```python
from build123d import *

# Parameters (mm, degrees)
EXTRUDE_1_DEPTH     = 4
SKETCH_2_R          = 1.1
CUT_EXTRUDE_1_DEPTH = 4
SKETCH_3_R          = 1.1
CUT_EXTRUDE_2_DEPTH = 5
FILLET_3_R          = 1


with BuildPart() as part:
    # 草图1 → 凸台-拉伸1 (new body)
    with BuildSketch(Plane(origin=(0, 0, 0), x_dir=(1, 0, 0), z_dir=(0, 1, 0))):
        with BuildLine():
            Line((-6.657117104, 10.234542642), (-6.657117104, 3.551431113))
            Line((-6.657117104, 3.551431113), (-4.657117104, 3.551431113))
            Line((-4.657117104, 3.551431113), (-4.657117104, 11.058134514))
            ThreePointArc((-4.657117104, 11.058134514), (-4.457117104, 16.10020126), (-4.257117104, 11.058134514))
            Line((-4.257117104, 11.058134514), (-4.257117104, 3.551431113))
            Line((-4.257117104, 3.551431113), (-2.257117104, 3.551431113))
            Line((-2.257117104, 3.551431113), (-2.257117104, 10.234542642))
            ThreePointArc((-2.257117104, 10.234542642), (-0.460935895, 13.749946041), (-2.557117104, 17.095144441))
            Line((-2.557117104, 17.095144441), (-2.557117104, 22.039302875))
            Line((-2.557117104, 22.039302875), (-6.357117104, 22.039302875))
            Line((-6.357117104, 22.039302875), (-6.357117104, 17.095144441))
            ThreePointArc((-6.357117104, 17.095144441), (-8.453298314, 13.749946041), (-6.657117104, 10.234542642))
        make_face()
    extrude(amount=EXTRUDE_1_DEPTH)

    # 草图2 → 切除-拉伸1 (cut)
    with BuildSketch(Plane(origin=(-2.457117104, 0, 0), x_dir=(0, 0, -1), z_dir=(1, 0, 0))):
        with Locations((20.139302875, 2)):
            Circle(SKETCH_2_R)
    extrude(amount=-CUT_EXTRUDE_1_DEPTH, mode=Mode.SUBTRACT)

    # 草图3 → 切除-拉伸2 (cut)
    with BuildSketch(Plane.ZY.offset(6.657117104)):
        with Locations((-6.551431113, 2)):
            Circle(SKETCH_3_R)
    extrude(amount=-CUT_EXTRUDE_2_DEPTH, mode=Mode.SUBTRACT)

    # 圆角3
    fillet_3_edges = [part.edges().sort_by_distance(p)[0] for p in [
        (-4.457117104, 4, -22.039302875),
        (-4.457117104, 0, -22.039302875),
    ]]
    fillet(fillet_3_edges, radius=FILLET_3_R)


solid = part.part
```
Verification items for the finished model (mm, model axes). A direction names the side the tool comes from. Give positions to 0.01 mm unless a question says otherwise; leave off trailing zeros. Order: outer loops, then holes, each group sorted by start corner. A loop starts at its lowest first (then second) coordinate and runs counter-clockwise, first axis right, second up. Notation, with made-up numbers: M 77,23 L 90,23 A28 cw 90,41 Z; hole C 22,-7 d5. An arc over 180 degrees is marked long. Answer in a Markdown table with one row per item. Add a question column.
Item 1: Section check A-A, the plane y = 2. Enter the section's corners in (x, z) (3 decimals), and give its area (3 significant figures).
Item 2: Mould release check, pull along Y, two halves, no side actions. Record for faces 1 (the cylindrical face through (-4.431, 1.579, -21.155)), 2 (the cylindrical face through (-5.671, 1.579, -5.535)), 3 (the flat face through (-5, 4, -10)), 4 (the flat face through (-6.357, 2, -18.5)): released by +Y, released by -Y, zero draft, split by the parting line, or undercut.
Item 3: Gauge pin test, flat ends, axial feed: pin 1 (1.8 mm diameter, centred on y = 2, z = -6.55, fed in from -X); pin 2 (1.5 mm diameter, centred on x = -7, z = -9.5, fed in from -Y); pin 3 (1.2 mm diameter, centred on y = 1.5, z = -6, fed in from -X); pin 4 (2 mm diameter, centred on y = 2, z = -19, fed in from -X). Record the tip position at first contact, or that the pin passes through.
Item 4: Scan lines: probe 1 along Z at (x, y) = (-3.75, 1.95); probe 2 along X at (y, z) = (3.1, -4.25); probe 3 along Y at (x, z) = (-3.5, -7). Record each from-to range of solid material in increasing order. Write a range as from..to.
Item 5: Section check C-C, the plane z = -6.5. Enter the section's corners in (x, y).
Item 6: Section check D-D, the plane z = -12.25. Enter the section's corners in (x, y), and give its area (3 significant figures).
Item 7: Tool access check on faces 5 (the flat face through (-4.657, 2, -8)), 6 (the flat face through (-6.657, 2, -8)), 7 (the cylindrical face through (-3.271, 1.579, -5.535)), 8 (the flat face through (-2.257, 2, -8)), 9 (the flat face through (-2.557, 1.53, -18.98)). Record the directions out of +Z, -Z, +X, -X, +Y, -Y that give a thin tool (end or side, any length) a straight path to the whole face; none if there is none.
Item 8: Section check B-B, the plane x = -3.25. Enter the section's corners in (y, z), and give its area (3 significant figures).
Filled sheet:
| question | item | result |
|---|---|---|
| 1 | outline | M -6.657,-10.235 A4 ccw -6.357,-17.095 L -6.357,-19.039 L -2.557,-19.039 L -2.557,-17.095 A4 ccw -2.257,-10.235 L -2.257,-7.651 L -4.257,-7.651 L -4.257,-11.058 A2.525 cw long -4.657,-11.058 L -4.657,-7.651 L -6.657,-7.651 Z; M -6.657,-5.451 L -4.657,-5.451 L -4.657,-3.551 L -6.657,-3.551 Z; M -6.357,-22.039 L -2.557,-22.039 L -2.557,-21.239 L -6.357,-21.239 Z; M -4.257,-5.451 L -2.257,-5.451 L -2.257,-3.551 L -4.257,-3.551 Z |
| 1 | area | 55.1 mm^2 |
| 2 | face 1 | undercut |
| 2 | face 2 | undercut |
| 2 | face 3 | released by +Y |
| 2 | face 4 | zero draft |
| 3 | pin 1 | passes through |
| 3 | pin 2 | stops at y = 0 |
| 3 | pin 3 | stops at x = -6.66 |
| 3 | pin 4 | stops at x = -6.36 |
| 4 | probe 1 | z = -22.04..-21.24, -19.04..-16, -11.15..-7.65, -5.45..-3.55 |
| 4 | probe 2 | x = -6.66..-4.66, -4.26..-2.26 |
| 4 | probe 3 | y = 0..1, 3..4 |
| 5 | outline | M -6.66,0 L -4.66,0 L -4.66,0.9 L -6.66,0.9 Z; M -6.66,3.1 L -4.66,3.1 L -4.66,4 L -6.66,4 Z; M -4.26,0 L -2.26,0 L -2.26,0.9 L -4.26,0.9 Z; M -4.26,3.1 L -2.26,3.1 L -2.26,4 L -4.26,4 Z |
| 6 | outline | M -8.23,0 L -6.61,0 L -6.61,4 L -8.23,4 Z; M -2.31,0 L -0.68,0 L -0.68,4 L -2.31,4 Z |
| 6 | area | 13.0 mm^2 |
| 7 | face 5 | +Z, +Y, -Y |
| 7 | face 6 | +Z, -X, +Y, -Y |
| 7 | face 7 | +X, -X |
| 7 | face 8 | +Z, +X, +Y, -Y |
| 7 | face 9 | -Z, +X, +Y, -Y |
| 8 | outline | M 0,-21.04 A1 ccw 1,-22.04 L 3,-22.04 A1 ccw 4,-21.04 L 4,-15.79 L 0,-15.79 Z; M 0,-11.36 L 4,-11.36 L 4,-3.55 L 0,-3.55 Z; hole C 2,-20.14 d2.2; hole C 2,-6.55 d2.2 |
| 8 | area | 48.2 mm^2 |
